```python
from build123d import *

# Parameters (mm, degrees)
PAD_DEPTH         = 14
POCKET_DEPTH      = 5.501
POCKET_DEPTH_BACK = 5.501
PAD001_DEPTH      = 17
PAD001_DEPTH_BACK = 15
SKETCH003_W       = 2.5
SKETCH003_H       = 4
PAD002_DEPTH      = 0.3


with BuildPart() as part:
    # Sketch → Pad (new body, symmetric)
    with BuildSketch(Plane.XY):
        with BuildLine():
            ThreePointArc((4.993006, 1.92728), (4.84786, 3.520957), (4.617941, 5.104626))
            ThreePointArc((4.617941, 5.104626), (4.065897, 6.174162), (3, 6.733201))
            ThreePointArc((3, 6.733201), (1.50592, 6.933169), (0, 7))
            Line((0, 7), (0, 0))
            Line((3.394019, 0), (0, 0))
            ThreePointArc((3.394019, 0), (4.783335, 0.56132), (5.3928, 1.930201))
            Line((5.3928, 1.930201), (5.5, 5))
            ThreePointArc((5.5, 5), (5.401745, 5.099985), (5.300061, 5.00349))
            Line((5.300061, 5.00349), (5.192739, 1.930201))
            ThreePointArc((4.993006, 1.92728), (5.094262, 1.833702), (5.192739, 1.930201))
        make_face()
    pad = extrude(amount=PAD_DEPTH, both=True)

    # Mirrored: Pad across Sketch V_Axis
    add(pad.mirror(Plane(origin=(0, 0, 0), x_dir=(0, 0, 1), z_dir=(1, 0, 0))))

    # Sketch001 → Pocket (cut, two sides)
    with BuildSketch(Plane.YZ) as pocket_sk:
        with BuildLine():
            Line((0, 14), (5.063511, 13.500005))
            ThreePointArc((6.866443, 11.555898), (6.333433, 12.869652), (5.063511, 13.500005))
            ThreePointArc((6.866443, -11.555898), (7, 0), (6.866443, 11.555898))
            ThreePointArc((5.063515, -13.499995), (6.333431, -12.869643), (6.866443, -11.555898))
            Line((5.063515, -13.499995), (0, -14))
            Line((0, -14), (0, -19))
            Line((0, -19), (10, -19))
            Line((10, -19), (10, 19))
            Line((10, 19), (0, 19))
            Line((0, 19), (0, 14))
        make_face()
    extrude(amount=-POCKET_DEPTH, mode=Mode.SUBTRACT)
    extrude(pocket_sk.sketch, amount=POCKET_DEPTH_BACK, mode=Mode.SUBTRACT)

    # Sketch002 → Pad001 (join, two sides)
    with BuildSketch(Plane.XY) as pad001_sk:
        with BuildLine():
            Line((5.3928, 1.930201), (5.5, 5))
            ThreePointArc((5.5, 5), (5.401745, 5.099985), (5.300061, 5.00349))
            Line((5.300061, 5.00349), (5.192739, 1.930201))
            ThreePointArc((3.394019, 0.193197), (4.644277, 0.698334), (5.192739, 1.930201))
            Line((0, 0.193197), (3.394019, 0.193197))
            Line((0, 0.193197), (0, 0))
            Line((3.394019, 0), (0, 0))
            ThreePointArc((3.394019, 0), (4.783335, 0.56132), (5.3928, 1.930201))
        make_face()
    pad001 = extrude(amount=PAD001_DEPTH) + extrude(pad001_sk.sketch, amount=-PAD001_DEPTH_BACK)

    # Mirrored001: Pad001 across Sketch002 V_Axis
    add(pad001.mirror(Plane(origin=(0, 0, 0), x_dir=(0, 0, 1), z_dir=(1, 0, 0))))

    # Sketch003 (on Face22 of Mirrored001) → Pad002 (join)
    with BuildSketch(Plane(origin=(0, 0.193197, 0), x_dir=(-1, 0, 0), z_dir=(0, 1, 0))):
        with Locations((-2.35, 15.2)):
            Rectangle(SKETCH003_W, SKETCH003_H)
        with Locations((2.35, 15.2)):
            Rectangle(SKETCH003_W, SKETCH003_H)
    extrude(amount=PAD002_DEPTH)


solid = part.part
```
The model under review builds one solid part; all positions refer to its coordinate system, in mm. A direction names the side the tool comes from. Give positions to 0.01 mm unless a question says otherwise; leave off trailing zeros. Write each loop counter-clockwise with the first axis right and the second up, starting at its lowest first coordinate (ties: lowest second). Pieces come first, ordered by that corner, then holes. Notation, with made-up numbers: M 50,-27 L 90,-27 A16 ccw 90,-4 Z; hole C 59,65 d2. An arc over 180 degrees is marked long. Write item = value, one per line. Start each with the question number.
Q1. We need section D-D (y = 1). State the section outline as (x, z) points.
Q2. Mouldability with a two-part tool opening along X and no side actions: class faces 5 (the face through (4.704, 0.759, 15.382)), 6 (the face through (-4.77, 0.55, 0.78)), 7 (the face through (0.03, 6.95, 6.98)), 8 (the face through (4.77, 0.55, 1.22)) as released by +X, released by -X, zero draft, split by the parting line, or undercut.
Q3. We need section A-A (y = 2.5). State the section outline as (x, z) points, plus the area to 3 significant figures.
Q4. For line 1 (X direction, y = 2, z = 13.5); line 2 (X direction, y = 2.75, z = 6.5); line 3 (Z direction, x = 1, y = 2), list the stretches that pass through material, from the lowest coordinate up.
Q5. We need section C-C (x = -1.5). State the section outline as (y, z) points.
Q6. Machinability: for faces 1 (the face through (-4.08, 6.16, 0.19)), 2 (the face through (0.073, 2.662, -13.737)), 3 (the face through (0, 0.193, 15)), 4 (the face through (-4.85, 3.5, 0.19)), which of the approach directions +Z, -Z, +X, -X, +Y, -Y give a long, thin tool a straight path to every point of the face, cutting with its end or side? Answer none if there is none.
Q7. We need section B-B (z = 11). State the section outline as (x, y) points, plus the area to 3 significant figures.
Q8. Clearance check with flat-ended pins moving along their axes: pin 1 (4 mm diameter, centred on x = 4, y = 5, fed in from -Z); pin 2 (1.2 mm diameter, centred on x = 2, z = 16, fed in from +Y); pin 3 (1.5 mm diameter, centred on x = 4, y = 6.5, fed in from -Z); pin 4 (2 mm diameter, centred on x = 2.5, z = 2, fed in from +Y). State where each tip first meets the part, or that it passes through.
Result set:
q1.outline = M -5.13,-15 L -4.9,-15 L -4.9,-13.9 L 4.9,-13.9 L 4.9,-15 L 5.13,-15 L 5.13,17 L 4.9,17 L 4.9,13.9 L -4.9,13.9 L -4.9,17 L -5.13,17 Z
q2.face_5 = undercut
q2.face_6 = released by -X
q2.face_7 = zero draft
q2.face_8 = released by +X
q3.outline = M -5.41,-15 L -5.21,-15 L -5.21,17 L -5.41,17 Z; M -4.95,-13.75 L 4.95,-13.75 L 4.95,13.75 L -4.95,13.75 Z; M 5.21,-15 L 5.41,-15 L 5.41,17 L 5.21,17 Z
q3.area = 285 mm2
q4.line_1 = -5.4 to -5.2, -4.99 to 4.99, 5.2 to 5.4
q4.line_2 = -5.42 to -5.22, -4.93 to 4.93, 5.22 to 5.42
q4.line_3 = -13.8 to 13.8
q5.outline = M 0,-15 L 0.19,-15 L 0.19,-13.98 L 5.06,-13.5 A2 ccw 6.87,-11.56 A500 ccw 6.93,-8.14 L 6.93,8.14 A500 ccw 6.87,11.56 A2 ccw 5.06,13.5 L 0.49,13.95 L 0.49,17.2 L 0.19,17.2 L 0.19,17 L 0,17 Z
q6.face_1 = +Z, -Z, -X, +Y
q6.face_2 = -Z, +Y
q6.face_3 = +Z, +Y
q6.face_4 = +Z, -Z, +Y
q7.outline = M -5.5,5 L -5.39,1.93 A2 ccw -3.39,0 L 3.39,0 A2 ccw 5.39,1.93 L 5.5,5 A0.1 ccw 5.3,5 L 5.19,1.93 A0.1 cw 4.99,1.93 A30 ccw 4.62,5.1 A2 ccw 3,6.73 A17 ccw 2.02,6.88 L -2.02,6.88 A17 ccw -3,6.73 A2 ccw -4.62,5.1 A30 ccw -4.99,1.93 A0.1 cw -5.19,1.93 L -5.3,5 A0.1 ccw Z
q7.area = 65.3 mm2
q8.pin_1 = -15
q8.pin_2 = 0.49
q8.pin_3 = -13.3
q8.pin_4 = 6.93
